Could you check a few things on this model? Use its own coordinates, in mm. A direction names the side the tool comes from. Give positions to 0.01 mm unless a question says otherwise; leave off trailing zeros. Order: outer loops, then holes, each group sorted by start corner. A loop starts at its lowest first (then second) coordinate and runs counter-clockwise, first axis right, second up. Notation, with made-up numbers: (14.5, -13) -> (53.5, -13) arc R18 cw to (53.5, -9) -> close; hole circle Ø4 at (7.25, 17.5). An arc over 180 degrees is marked (long way). One line per item, written item: value.
```python
from build123d import *

# Parameters (mm, degrees)
F1_DEPTH      = 17.5
F1_DEPTH_BACK = 17.5
F2_SIZE       = 15
F3_SIZE       = 7.5
F5_W          = 3
F5_H          = 92.5
F6_DEPTH      = 0.01
F7_W          = 3
F7_H          = 92.5
F8_DEPTH      = 0.01
F4_R          = 2.1
F9_DEPTH      = 3
F11_DEPTH     = 10
F13_DEPTH     = 10


with BuildPart() as f1:
    # F0 (on Top) → F1 (new body, two sides)
    with BuildSketch(Plane.XY) as f1_sk:
        Polygon((147.5, -50), (147.5, 50), (-147.5, 50), (-147.5, -50), (-144.5, -50), (-144.5, -30), (144.5, -30), (144.5, -50), align=None)
    extrude(amount=F1_DEPTH)
    extrude(f1_sk.sketch, amount=-F1_DEPTH_BACK)

    # F2
    f2_edges = [f1.edges().sort_by_distance(p)[0] for p in [
        (0, -30, 17.5),
        (0, -30, -17.5),
    ]]
    chamfer(f2_edges, length=F2_SIZE)

    # F3
    f3_edges = [f1.edges().sort_by_distance(p)[0] for p in [
        (146, -50, 17.5),
        (146, -50, -17.5),
        (-146, -50, 17.5),
        (-146, -50, -17.5),
    ]]
    chamfer(f3_edges, length=F3_SIZE)

    # F5 (on face) → F6 (join)
    with BuildSketch(Plane.XY.offset(17.5)):
        with Locations((-146, 3.75)):
            Rectangle(F5_W, F5_H)
        with Locations((146, 3.75)):
            Rectangle(F5_W, F5_H)
    extrude(amount=F6_DEPTH)

    # F7 (on face) → F8 (join)
    with BuildSketch(Plane(origin=(0, 0, -17.5), x_dir=(1, 0, 0), z_dir=(0, 0, -1))):
        with Locations((-146, -3.75)):
            Rectangle(F7_W, F7_H)
        with Locations((146, -3.75)):
            Rectangle(F7_W, F7_H)
    extrude(amount=F8_DEPTH)

    # F4 (on face) → F9 (cut)
    with BuildSketch(Plane.YZ.offset(147.5)):
        with BuildLine():
            ThreePointArc((47.5, 0), (46.767767, 1.767767), (45, 2.5))
            Line((45, 2.5), (25, 2.5))
            ThreePointArc((25, 2.5), (23.232233, 1.767767), (22.5, 0))
            ThreePointArc((22.5, 0), (23.232233, -1.767767), (25, -2.5))
            Line((25, -2.5), (45, -2.5))
            ThreePointArc((45, -2.5), (46.767767, -1.767767), (47.5, 0))
        make_face()
        with Locations((35, 0)):
            Circle(F4_R, mode=Mode.SUBTRACT)
        with BuildLine():
            ThreePointArc((7.5, 0), (6.767767, 1.767767), (5, 2.5))
            Line((5, 2.5), (-15, 2.5))
            ThreePointArc((-15, 2.5), (-16.767767, 1.767767), (-17.5, 0))
            ThreePointArc((-17.5, 0), (-16.767767, -1.767767), (-15, -2.5))
            Line((-15, -2.5), (5, -2.5))
            ThreePointArc((5, -2.5), (6.767767, -1.767767), (7.5, 0))
        make_face()
        with Locations((-5, 0)):
            Circle(F4_R, mode=Mode.SUBTRACT)
    extrude(amount=-F9_DEPTH, mode=Mode.SUBTRACT)

    # F10 (on face) → F11 (cut)
    with BuildSketch(Plane.XY.offset(17.5)):
        with BuildLine():
            Line((139.5, 50), (-139.5, 50))
            Line((-139.5, 50), (-139.5, 0))
            ThreePointArc((-139.5, 0), (-136.571068, -7.071068), (-129.5, -10))
            Line((-129.5, -10), (129.5, -10))
            ThreePointArc((129.5, -10), (136.571068, -7.071068), (139.5, 0))
            Line((139.5, 0), (139.5, 50))
        make_face()
    extrude(amount=-F11_DEPTH, mode=Mode.SUBTRACT)

    # F12 (on face) → F13 (cut)
    with BuildSketch(Plane(origin=(0, 0, -17.5), x_dir=(1, 0, 0), z_dir=(0, 0, -1))):
        with BuildLine():
            Line((139.5, -50), (139.5, 0))
            ThreePointArc((139.5, 0), (136.571068, 7.071068), (129.5, 10))
            Line((129.5, 10), (-129.5, 10))
            ThreePointArc((-129.5, 10), (-136.571068, 7.071068), (-139.5, 0))
            Line((-139.5, 0), (-139.5, -50))
            Line((-139.5, -50), (139.5, -50))
        make_face()
    extrude(amount=-F13_DEPTH, mode=Mode.SUBTRACT)


solid = f1.part
```
1) Suppose I cut it at C-C, the plane y = -20.5. Write out the boundary of the cut face in (x, z).
Answer below:
outline: (-147.5, -17.51) -> (-144.5, -17.51) -> (-144.5, -12) -> (144.5, -12) -> (144.5, -17.51) -> (147.5, -17.51) -> (147.5, 17.51) -> (144.5, 17.51) -> (144.5, 12) -> (-144.5, 12) -> (-144.5, 17.51) -> (-147.5, 17.51) -> close
2) Suppose I cut it at B-B, the plane x = -13. Write out the boundary of the cut face in (y, z), then the cut area to 4 significant figures.
Answer below:
outline: (-30, -2.5) -> (-15, -17.5) -> (-10, -17.5) -> (-10, -7.5) -> (50, -7.5) -> (50, 7.5) -> (-10, 7.5) -> (-10, 17.5) -> (-15, 17.5) -> (-30, 2.5) -> close
area: 1,375 mm2
3) We'd pull the mould along X, two halves only. Please class faces 6 (the flat face through (144.5, -5.2, 2.3)), 7 (the cylindrical face through (-136.65, -6.99, 12.57)), 8 (the flat face through (-146, -46, -14)): +X half, -X half, draft (parallel to the pull), parting line (faces both ways), or undercut.
Answer below:
face 6: +X half
face 7: undercut
face 8: draft
4) For faces 1 (the flat face through (-2, -22.4, -10.1)), 2 (the cylindrical face through (136.49, -7.15, 12.57)), 3 (the flat face through (144.5, -37, 0)), 4 (the flat face through (139.5, 25, -13)), 5 (the flat face through (-2, -30, 0)), which set-ups out of +Z, -Z, +X, -X, +Y, -Y let a thin tool reach every point of the face, with its end or its side?
Answer below:
face 1: -Z, -Y
face 2: +Z, +Y
face 3: -Y
face 4: -Z, +Y
face 5: +Z, -Z, -Y
5) For P1, Ø5, axis at x = -63.5, y = -19.5, coming from the +Z side; P2, Ø1.5, axis at x = 4.5, z = 10.5, coming from the +Y side; P3, Ø2, axis at x = -81.5, y = 1, coming from the -Z side, each with a flat end and sliding along its axis, tell me the tip position at first contact or that it passes through.
Answer below:
P1: stops at z = 15.5
P2: stops at y = -10
P3: stops at z = -7.5
6) If I drill on line 1 along X through (y, z) = (2.5, 10.5); line 2 along X through (y, z) = (-35.5, 5); line 3 along Y through (x, z) = (30.5, 1), over which ranges is the centre line in solid material (lowest first)?
Answer below:
line 1: x = -147.5 to -139.5, 139.5 to 147.5
line 2: x = -147.5 to -144.5, 144.5 to 147.5
line 3: y = -30 to 50
